Here's how the part is built. I have some questions about the finished solid (model axes, mm). Face numbers are marked on the shaded views. A direction names the side the tool comes from. Coordinates: 2 decimals unless noted, no trailing zeros. Order: outer loops, then holes, each group sorted by start corner. A loop starts at its lowest first (then second) coordinate and runs counter-clockwise, first axis right, second up. Notation, with made-up numbers: (24, 27.5) - (72, 27.5) arc R17 cw to (72, 40.5) - close; hole circle Ø10 at (25, 38). An arc over 180 degrees is marked (long way). Answer in a Markdown table with one row per item. Add a question column.
Item 1: I want a section at A-A (z = 6.75). Please give me the cut outline in (x, y), plus the area to 3 significant figures.
Item 2: I want a section at B-B (y = 28.5). Please give me the cut outline in (x, z).
Item 3: I want a section at C-C (x = -4.75). Please give me the cut outline in (y, z), plus the area to 3 significant figures.
Item 4: Thinking about a two-plate mould opening in X: for the marked faces 1, 2 and 3, which applies, +X half, -X half, draft (parallel to the pull), parting line (faces both ways), or undercut?
Item 5: If I drill on line 1 along Y through (x, z) = (8, 1.15); line 2 along Y through (x, z) = (-8, 2.3); line 3 along Y through (x, z) = (-0.5, 3.5), over which ranges is the centre line in solid material (lowest first)? Write a range as from..to.
Item 6: Will these pins go through, and if not, where does the flat tip stop? pin 1 Ø5 at (x, y) = (-8, 42) entering from +Z; pin 2 Ø1 at (x, z) = (7.5, 6) entering from -Y; pin 3 Ø7 at (x, y) = (5.5, -23.5) entering from +Z.
Item 7: On a 3-axis mill with a long thin cutter (end or side, diameter ignored), from which of +Z, -Z, +X, -X, +Y, -Y can I reach the whole of each face in a straight line? I mean the marked faces 4, 5 and 6. Say none if no direction works.
```python
from build123d import *

# Parameters (mm, degrees)
F1_DEPTH = 2
F2_DEPTH = 18
F0_R     = 0.5
F3_DEPTH = 3


with BuildPart() as f1:
    # F0 (on Top) → F1 (new body)
    with BuildSketch(Plane.XY):
        Polygon((-3, 54.44269), (-9.5, 54.44269), (-9.5, -13.55731), (-3, -13.55731), (-3, -12.75731), (0, -12.75731), (3, -12.75731), (3, -13.55731), (9.5, -13.55731), (9.5, 54.44269), (3, 54.44269), (3, 53.64269), (0, 53.64269), (-3, 53.64269), align=None)
    extrude(amount=F1_DEPTH)

    # F0 (on Top) → F2 (join)
    with BuildSketch(Plane.XY):
        Polygon((-11.5, -15.55731), (0, -15.55731), (11.5, -15.55731), (11.5, 56.44269), (0, 56.44269), (-11.5, 56.44269), align=None)
        Polygon((-9.5, -13.55731), (-9.5, 54.44269), (-3, 54.44269), (0, 54.44269), (3, 54.44269), (9.5, 54.44269), (9.5, -13.55731), (3, -13.55731), (0, -13.55731), (-3, -13.55731), align=None, mode=Mode.SUBTRACT)
    extrude(amount=F2_DEPTH)

    # F0 (on Top) → F3 (join)
    with BuildSketch(Plane.XY):
        Polygon((11.5, -15.55731), (0, -15.55731), (-11.5, -15.55731), (-11.5, -40.55731), (0, -40.55731), (11.5, -40.55731), align=None)
        with Locations((-8, -39.05731)):
            Circle(F0_R, mode=Mode.SUBTRACT)
        with Locations((-8, -17.05731)):
            Circle(F0_R, mode=Mode.SUBTRACT)
        with Locations((8, -39.05731)):
            Circle(F0_R, mode=Mode.SUBTRACT)
        with Locations((8, -17.05731)):
            Circle(F0_R, mode=Mode.SUBTRACT)
    extrude(amount=F3_DEPTH)


solid = f1.part
```
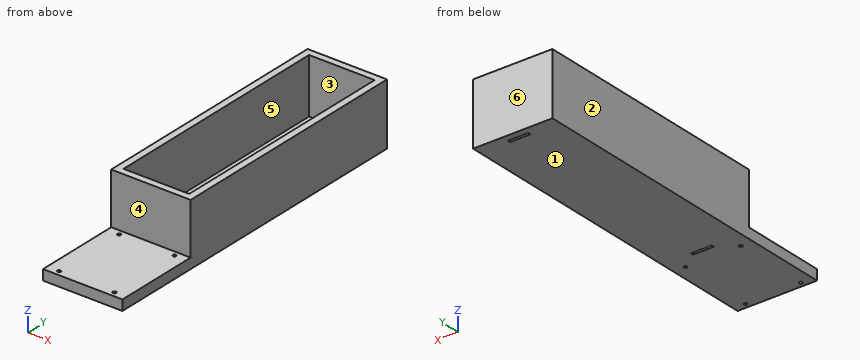
Values follow:
| question | item | result |
|---|---|---|
| 1 | outline | (-11.5, -15.56) - (11.5, -15.56) - (11.5, 56.44) - (-11.5, 56.44) - close; hole (-9.5, -13.56) - (9.5, -13.56) - (9.5, 54.44) - (-9.5, 54.44) - close |
| 1 | area | 364 mm^2 |
| 2 | outline | (-11.5, 0) - (11.5, 0) - (11.5, 18) - (9.5, 18) - (9.5, 2) - (-9.5, 2) - (-9.5, 18) - (-11.5, 18) - close |
| 3 | outline | (-40.56, 0) - (56.44, 0) - (56.44, 18) - (54.44, 18) - (54.44, 2) - (-13.56, 2) - (-13.56, 18) - (-15.56, 18) - (-15.56, 3) - (-40.56, 3) - close |
| 3 | area | 283 mm^2 |
| 4 | face 1 | draft |
| 4 | face 2 | -X half |
| 4 | face 3 | undercut |
| 5 | line 1 | y = -40.56..-39.56, -38.56..-17.56, -16.56..56.44 |
| 5 | line 2 | y = -40.56..-39.56, -38.56..-17.56, -16.56..-13.56, 54.44..56.44 |
| 5 | line 3 | y = -15.56..-13.56, 54.44..56.44 |
| 6 | pin 1 | stops at z = 18 |
| 6 | pin 2 | stops at y = -15.56 |
| 6 | pin 3 | stops at z = 3 |
| 7 | face 4 | +Z, +X, -X, -Y |
| 7 | face 5 | +Z |
| 7 | face 6 | +Z, -Z, +X, -X, +Y |
